Part model, mm, in its own coordinate system. A direction names the side the tool comes from. Coordinates: 2 decimals unless noted, no trailing zeros. Loops run counter-clockwise (first coordinate to the right, second up) from the corner with the lowest first, then second, coordinate; pieces in that order, holes last. Notation, with made-up numbers: (53.5, -40) -> (59.5, -40) arc R26 ccw to (59.5, -2) -> close; hole circle Ø4 at (88, -31.75). An arc over 180 degrees is marked (long way). Use one line per item in the form item = value. Start each with the question number.
(1) 3-axis set-ups, long thin cutter, end or side, ignore diameter. For faces 1 (the flat face through (30, -11, 0)), 2 (the cylindrical face through (0, -25, -1)): which of +Z, -Z, +X, -X, +Y, -Y reach the whole face in a straight line?
(2) Drill centre lines: L1, parallel to Y at x = -7, z = 4.5; L2, parallel to Z at x = 0, y = -25; L3, parallel to Z at x = 0, y = -25.25. Where is each one in solid material? Low to high. Write a range as [from, to].
(3) Band-saw the part on A-A on z = 27. Give the cut face in (x, y).
(4) Band-saw the part on D-D on y = -3.5. Give the cut face in (x, z), then the cut area to 4 significant figures.
(5) Band-saw the part on C-C on z = 0. Give the cut face in (x, y), then the cut area to 3 significant figures.
(6) Pin check, flat tips, straight feed: P1, Ø1, axis at x = 22, y = -16.5, coming from the +Z side; P2, Ø5, axis at x = 6.5, z = -17, coming from the -Y side; P3, Ø2, axis at x = 0, z = 0.5, coming from the -Y side; P4, Ø5, axis at y = -11, z = -23, coming from the +X side. Stop position of each tip, or through.
(7) Mould opens along Z. For faces 3 (the flat face through (-1, 5, 0)), 4 (the flat face through (0, 2, -35)), 5 (the flat face through (-30, -11, 0)), 6 (the flat face through (0, -24, 0)) say: +Z half, -Z half, draft (parallel to the pull), parting line (faces both ways), or undercut.
(8) Band-saw the part on B-B on x = 17. Give the cut face in (y, z).
```python
from build123d import *

# Parameters (mm, degrees)
F0_W     = 80
F0_H     = 70
F1_DEPTH = 26
F2_SIZE  = 25
F3_DEPTH = 5
F4_R     = 5
F5_W     = 75
F5_H     = 65
F6_DEPTH = 1
F7_R     = 1
F8_DEPTH = 2


with BuildPart() as f1:
    # F0 (on Front) → F1 (new body)
    with BuildSketch(Plane.XZ):
        Rectangle(F0_W, F0_H)
    extrude(amount=F1_DEPTH)

    # F2
    f2_edges = [f1.edges().sort_by_distance(p)[0] for p in [
        (0, -26, -35),
        (40, -26, 0),
        (0, -26, 35),
        (-40, -26, 0),
    ]]
    chamfer(f2_edges, length=F2_SIZE)

    # F3 (add): a face of the model
    f3_faces = [f1.faces().sort_by_distance(p)[0] for p in [
        (0, 0, 0),
    ]]
    extrude(f3_faces, amount=F3_DEPTH)

    # F4
    f4_edges = [f1.edges().sort_by_distance(p)[0] for p in [
        (40, 2, 35),
        (-40, 2, 35),
        (40, 2, -35),
        (-40, 2, -35),
    ]]
    fillet(f4_edges, radius=F4_R)

    # F5 (on face) → F6 (join)
    with BuildSketch(Plane(origin=(0, 5, 0), x_dir=(-1, 0, 0), z_dir=(0, 1, 0))):
        with BuildLine():
            ThreePointArc((-40, -30), (-38.5355339059, -33.5355339059), (-35, -35))
            Line((-35, -35), (35, -35))
            ThreePointArc((35, -35), (38.5355339059, -33.5355339059), (40, -30))
            Line((40, -30), (40, 30))
            ThreePointArc((40, 30), (38.5355339059, 33.5355339059), (35, 35))
            Line((35, 35), (-35, 35))
            ThreePointArc((-35, 35), (-38.5355339059, 33.5355339059), (-40, 30))
            Line((-40, 30), (-40, -30))
        make_face()
        Rectangle(F5_W, F5_H, mode=Mode.SUBTRACT)
    extrude(amount=F6_DEPTH)

    # F7 (on face) → F8 (cut)
    with BuildSketch(Plane.XZ.offset(26)):
        Circle(F7_R)
    extrude(amount=-F8_DEPTH, mode=Mode.SUBTRACT)


solid = f1.part
```
A:
q1.face_1 = +Z, -Z, +X, -Y
q1.face_2 = -Y
q2.L1 = [-26, 5]
q2.L2 = [-11, -1], [1, 11]
q2.L3 = [-10.75, -1], [1, 10.75]
q3.outline = (-40, -1) -> (-32, -9) -> (32, -9) -> (40, -1) -> (40, 6) -> (37.5, 6) -> (37.5, 5) -> (-37.5, 5) -> (-37.5, 6) -> (-40, 6) -> close
q4.outline = (-37.5, -32.5) -> (37.5, -32.5) -> (37.5, 32.5) -> (-37.5, 32.5) -> close
q4.area = 4,875 mm²
q5.outline = (-40, -1) -> (-15, -26) -> (-1, -26) -> (-1, -24) -> (1, -24) -> (1, -26) -> (15, -26) -> (40, -1) -> (40, 6) -> (37.5, 6) -> (37.5, 5) -> (-37.5, 5) -> (-37.5, 6) -> (-40, 6) -> close
q5.area = 1,860 mm²
q6.P1 = 20
q6.P2 = -21.5
q6.P3 = -26
q6.P4 = 32.5
q7.face_3 = undercut
q7.face_4 = -Z half
q7.face_5 = draft
q7.face_6 = undercut
q8.outline = (-24, -12) -> (-1, -35) -> (6, -35) -> (6, -32.5) -> (5, -32.5) -> (5, 32.5) -> (6, 32.5) -> (6, 35) -> (-1, 35) -> (-24, 12) -> close
